Design review of the part built by this model. Coordinates are the model's own, in mm. A direction names the side the tool comes from. Coordinates: 2 decimals unless noted, no trailing zeros. Loops run counter-clockwise (first coordinate to the right, second up) from the corner with the lowest first, then second, coordinate; pieces in that order, holes last. Notation, with made-up numbers: (43.25, -33.5) - (79.25, -33.5) arc R31 cw to (79.25, -6.5) - close; hole circle Ø4 at (59.25, 89.5). An arc over 180 degrees is marked (long way). Answer in a Markdown table with one row per item. Add a question column.
(1) Clearance check with flat-ended pins moving along their axes: pin 1 (5 mm diameter, centred on x = 0.5, z = 0.5, fed in from +Y) (3 decimals); pin 2 (4 mm diameter, centred on x = -12, z = -4, fed in from +Y). State where each tip first meets the part, or that it passes through.
(2) To check wall thickness, follow L1, parallel to Z at x = -1.5, y = 1.3; L2, parallel to X at y = 1.3, z = -14; L3, parallel to Y at x = 13, z = -17. State the ranges of each line that lie inside material, in increasing order. Write a range as [from, to].
(3) We need section A-A, the plane z = -17. Write out the cut boundary in (x, y).
(4) We need section D-D, the plane x = -14. Write out the cut boundary in (y, z), plus the area to 3 significant figures.
(5) The part is to be moulded in two halves that separate along Z. For faces 1 (the face through (-16, 1.5, -2)), 2 (the face through (0, 1.125, 1)), 3 (the face through (0, 1, 22.5)), say which applies: released by +Z, released by -Z, zero draft, split by the parting line, or undercut.
(6) We need section C-C, the plane z = 3.5. Write out the cut boundary in (x, y) (3 decimals), plus the area to 3 significant figures.
(7) For faces 4 (the face through (-10, 1, 0)), 5 (the face through (17.5, 1, 0)), list the 3-axis set-ups (+Z, -Z, +X, -X, +Y, -Y) from which the entire face can be reached by the end or side of a thin tool; tool diameter is ignored.
(8) We need section B-B, the plane x = 7. Write out the cut boundary in (y, z) (3 decimals).
from build123d import *

# Parameters (mm, degrees)
SKETCH1_W           = 35
SKETCH1_H           = 45
BOSS_EXTRUDE1_DEPTH = 1.5
SKETCH2_W           = 30
SKETCH2_H           = 40
CUT_EXTRUDE1_DEPTH  = 0.5
BOSS_EXTRUDE2_DEPTH = 0.125


with BuildPart() as part:
    # Sketch1 → Boss-Extrude1 (new body)
    with BuildSketch(Plane(origin=(0, 0, 0), x_dir=(1, 0, 0), z_dir=(0, 1, 0))):
        Rectangle(SKETCH1_W, SKETCH1_H)
    extrude(amount=BOSS_EXTRUDE1_DEPTH)

    # Sketch2 → Cut-Extrude1 (cut)
    with BuildSketch(Plane(origin=(0, 1.5, 0), x_dir=(1, 0, 0), z_dir=(0, 1, 0))):
        Rectangle(SKETCH2_W, SKETCH2_H)
    extrude(amount=-CUT_EXTRUDE1_DEPTH, mode=Mode.SUBTRACT)

    # Sketch3 → Boss-Extrude2 (add)
    with BuildSketch(Plane(origin=(0, 1, 0), x_dir=(1, 0, 0), z_dir=(0, 1, 0))):
        with BuildLine():
            Line((-1.5, -10.5), (-1.5, -18))
            ThreePointArc((-1.5, -18), (-1.353553391, -18.353553391), (-1, -18.5))
            Line((-1, -18.5), (-0.5, -18.5))
            Line((-0.5, -18.5), (-0.5, -20))
            Line((-0.5, -20), (0.5, -20))
            Line((0.5, -20), (0.5, -18.5))
            Line((0.5, -18.5), (1, -18.5))
            ThreePointArc((1, -18.5), (1.353553391, -18.353553391), (1.5, -18))
            Line((1.5, -18), (1.5, -10.5))
            ThreePointArc((1.5, -10.5), (1.646446609, -10.146446609), (2, -10))
            Line((2, -10), (7.5, -10))
            ThreePointArc((7.5, -10), (7.853553391, -9.853553391), (8, -9.5))
            Line((8, -9.5), (8, 9.5))
            ThreePointArc((8, 9.5), (7.853553391, 9.853553391), (7.5, 10))
            Line((7.5, 10), (-7.5, 10))
            ThreePointArc((-7.5, 10), (-7.853553391, 9.853553391), (-8, 9.5))
            Line((-8, 9.5), (-8, -9.5))
            ThreePointArc((-8, -9.5), (-7.853553391, -9.853553391), (-7.5, -10))
            Line((-7.5, -10), (-2, -10))
            ThreePointArc((-2, -10), (-1.646446609, -10.146446609), (-1.5, -10.5))
        make_face()
    extrude(amount=BOSS_EXTRUDE2_DEPTH)


solid = part.part
Responses:
| question | item | result |
|---|---|---|
| 1 | pin 1 | stops at y = 1.125 |
| 1 | pin 2 | stops at y = 1 |
| 2 | L1 | z = [-22.5, -20], [20, 22.5] |
| 2 | L2 | x = [-17.5, -15], [15, 17.5] |
| 2 | L3 | y = [0, 1] |
| 3 | outline | (-17.5, 0) - (17.5, 0) - (17.5, 1.5) - (15, 1.5) - (15, 1) - (-15, 1) - (-15, 1.5) - (-17.5, 1.5) - close |
| 4 | outline | (0, -22.5) - (1.5, -22.5) - (1.5, -20) - (1, -20) - (1, 20) - (1.5, 20) - (1.5, 22.5) - (0, 22.5) - close |
| 4 | area | 47.5 mm2 |
| 5 | face 1 | zero draft |
| 5 | face 2 | undercut |
| 5 | face 3 | released by +Z |
| 6 | outline | (-17.5, 0) - (17.5, 0) - (17.5, 1.5) - (15, 1.5) - (15, 1) - (8, 1) - (8, 1.125) - (-8, 1.125) - (-8, 1) - (-15, 1) - (-15, 1.5) - (-17.5, 1.5) - close |
| 6 | area | 39.5 mm2 |
| 7 | face 4 | +Y |
| 7 | face 5 | +Z, -Z, +X, +Y, -Y |
| 8 | outline | (0, -22.5) - (1.5, -22.5) - (1.5, -20) - (1, -20) - (1, -10) - (1.125, -10) - (1.125, 10) - (1, 10) - (1, 20) - (1.5, 20) - (1.5, 22.5) - (0, 22.5) - close |
